Study the drawing (mm; zero at the part's minimum x, y, z) and answer. Coordinates: 2 decimals unless noted, no trailing zeros. Order: outer loops, then holes, each group sorted by start corner. A loop starts at its lowest first (then second) coordinate and runs counter-clockwise, first axis right, second up. Notation, with made-up numbers: (-25, 70.5) -> (-6, 70.5) arc R9 ccw to (-6, 84.5) -> close; hole circle Ø4 at (17, 24). An arc over 180 degrees is marked (long way). Answer as CSV lines item,"result". Start each with the question number.
Item 1: Straight lines are drawn through the part: L1, parallel to X at y = 1.15, z = 9.5; L2, parallel to Z at x = 64.5, y = 0.2; L3, parallel to Z at x = 49.5, y = 0.6. For each, find the intervals that lie inside material, in ascending order.
Item 2: Section B-B (z = 9.5) is taken. Write down the section's boundary in (x, y), then the cut area to 3 significant figures.
Item 3: Section A-A (x = 44) is taken. Write down the section's boundary in (y, z).
Item 4: Section D-D (x = 62) is taken. Write down the section's boundary in (y, z).
Item 5: Section C-C (y = 1.3) is taken. Write down the section's boundary in (x, z).
Item 6: Each of these flat-tipped pins is pushed along its axis until it touches: pin 1 Ø4 at (x, z) = (26, 9.5) entering from +Y; pin 2 Ø0.5 at (x, y) = (15, 0.5) entering from -Z; pin 3 Ø3 at (x, z) = (50.5, 5) entering from -Y (3 decimals); pin 4 Ø0.8 at (y, z) = (0.5, 1.5) entering from +X. Where does it stop, or does it pass through?
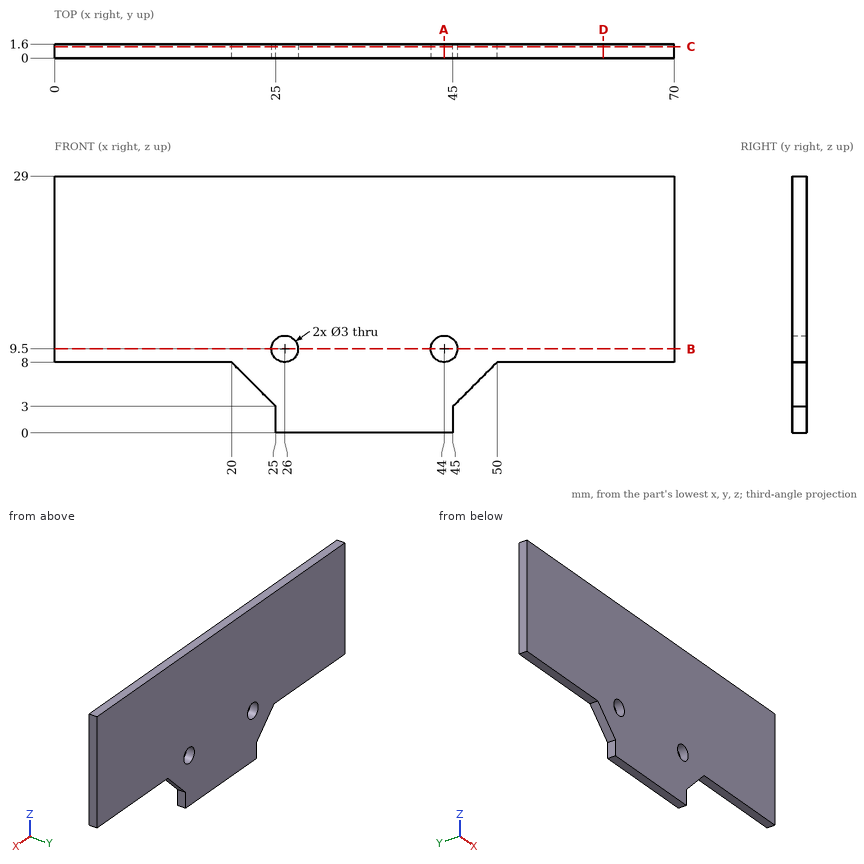
Checked values:
1,L1,"x = 0 to 24.5, 27.5 to 42.5, 45.5 to 70"
1,L2,"z = 8 to 29"
1,L3,"z = 7.5 to 29"
2,outline,"(0, 0) -> (24.5, 0) -> (24.5, 1.6) -> (0, 1.6) -> close; (27.5, 0) -> (42.5, 0) -> (42.5, 1.6) -> (27.5, 1.6) -> close; (45.5, 0) -> (70, 0) -> (70, 1.6) -> (45.5, 1.6) -> close"
2,area,"102 mm^2"
3,outline,"(0, 0) -> (1.6, 0) -> (1.6, 8) -> (0, 8) -> close; (0, 11) -> (1.6, 11) -> (1.6, 29) -> (0, 29) -> close"
4,outline,"(0, 8) -> (1.6, 8) -> (1.6, 29) -> (0, 29) -> close"
5,outline,"(0, 8) -> (20, 8) -> (25, 3) -> (25, 0) -> (45, 0) -> (45, 3) -> (50, 8) -> (70, 8) -> (70, 29) -> (0, 29) -> close; hole circle Ø3 at (26, 9.5); hole circle Ø3 at (44, 9.5)"
6,pin 1,"stops at y = 1.6"
6,pin 2,"stops at z = 8"
6,pin 3,"passes through"
6,pin 4,"stops at x = 45"
